Work out the finished part from the listing and answer in its coordinate system (mm). A direction names the side the tool comes from. Round coordinates to 2 decimals unless told otherwise and drop trailing zeros. Write each loop counter-clockwise with the first axis right and the second up, starting at its lowest first coordinate (ties: lowest second). Pieces come first, ordered by that corner, then holes. Notation, with made-up numbers: (-9.75, 48) -> (33.25, 48) arc R28 ccw to (33.25, 82) -> close; hole circle Ø6 at (78.5, 42.25). An arc over 180 degrees is marked (long way). One line per question, with ' | ' between items. Start each with the question number.
```python
from build123d import *

# Parameters (mm, degrees)
F0_W     = 350
F0_H     = 350
F1_DEPTH = 16
F2_DEPTH = 3
F3_W     = 350
F3_H     = 350
F3_W_2   = 318
F3_H_2   = 318
F4_DEPTH = 5
F5_R     = 1


with BuildPart() as f1:
    # F0 (on Front) → F1 (new body)
    with BuildSketch(Plane.XZ):
        with Locations((7.3111886159, -13.1394357215)):
            Rectangle(F0_W, F0_H)
        with BuildLine():
            ThreePointArc((-127.6888113841, 89.8605642785), (-118.3162283821, 112.4879812765), (-95.6888113841, 121.8605642785))
            Line((-95.6888113841, 121.8605642785), (110.3111886159, 121.8605642785))
            ThreePointArc((110.3111886159, 121.8605642785), (132.9386056138, 112.4879812765), (142.3111886159, 89.8605642785))
            Line((142.3111886159, 89.8605642785), (142.3111886159, -116.1394357215))
            ThreePointArc((142.3111886159, -116.1394357215), (132.9386056138, -138.7668527195), (110.3111886159, -148.1394357215))
            Line((110.3111886159, -148.1394357215), (-95.6888113841, -148.1394357215))
            ThreePointArc((-95.6888113841, -148.1394357215), (-118.3162283821, -138.7668527195), (-127.6888113841, -116.1394357215))
            Line((-127.6888113841, -116.1394357215), (-127.6888113841, 89.8605642785))
        make_face(mode=Mode.SUBTRACT)
    extrude(amount=F1_DEPTH)

    # F0 (on Front) → F2 (join)
    with BuildSketch(Plane.XZ):
        with Locations((7.3111886159, -13.1394357215)):
            Rectangle(F0_W, F0_H)
        with BuildLine():
            ThreePointArc((-127.6888113841, 89.8605642785), (-118.3162283821, 112.4879812765), (-95.6888113841, 121.8605642785))
            Line((-95.6888113841, 121.8605642785), (110.3111886159, 121.8605642785))
            ThreePointArc((110.3111886159, 121.8605642785), (132.9386056138, 112.4879812765), (142.3111886159, 89.8605642785))
            Line((142.3111886159, 89.8605642785), (142.3111886159, -116.1394357215))
            ThreePointArc((142.3111886159, -116.1394357215), (132.9386056138, -138.7668527195), (110.3111886159, -148.1394357215))
            Line((110.3111886159, -148.1394357215), (-95.6888113841, -148.1394357215))
            ThreePointArc((-95.6888113841, -148.1394357215), (-118.3162283821, -138.7668527195), (-127.6888113841, -116.1394357215))
            Line((-127.6888113841, -116.1394357215), (-127.6888113841, 89.8605642785))
        make_face(mode=Mode.SUBTRACT)
        with BuildLine():
            Line((110.3111886159, 121.8605642785), (-95.6888113841, 121.8605642785))
            ThreePointArc((-95.6888113841, 121.8605642785), (-118.3162283821, 112.4879812765), (-127.6888113841, 89.8605642785))
            Line((-127.6888113841, 89.8605642785), (-127.6888113841, -116.1394357215))
            ThreePointArc((-127.6888113841, -116.1394357215), (-118.3162283821, -138.7668527195), (-95.6888113841, -148.1394357215))
            Line((-95.6888113841, -148.1394357215), (110.3111886159, -148.1394357215))
            ThreePointArc((110.3111886159, -148.1394357215), (132.9386056138, -138.7668527195), (142.3111886159, -116.1394357215))
            Line((142.3111886159, -116.1394357215), (142.3111886159, 89.8605642785))
            ThreePointArc((142.3111886159, 89.8605642785), (132.9386056138, 112.4879812765), (110.3111886159, 121.8605642785))
        make_face()
    extrude(amount=-F2_DEPTH)

    # F3 (on face) → F4 (join)
    with BuildSketch(Plane(origin=(0, 3, 0), x_dir=(-1, 0, 0), z_dir=(0, 1, 0))):
        with Locations((-7.3111886159, -13.1394357215)):
            Rectangle(F3_W, F3_H)
        with Locations((-7.3111886159, -13.1394357215)):
            Rectangle(F3_W_2, F3_H_2, mode=Mode.SUBTRACT)
    extrude(amount=F4_DEPTH)

    # F5
    f5_edges = [f1.edges().sort_by_distance(p)[0] for p in [
        (7.311189, -16, 161.860564),
        (-167.688811, -16, -13.139436),
        (7.311189, -16, -188.139436),
        (182.311189, -16, -13.139436),
        (-118.316228, -16, 112.487981),
        (7.311189, -16, 121.860564),
        (132.938606, -16, 112.487981),
        (142.311189, -16, -13.139436),
        (132.938606, -16, -138.766853),
        (7.311189, -16, -148.139436),
        (-118.316228, -16, -138.766853),
        (-127.688811, -16, -13.139436),
    ]]
    fillet(f5_edges, radius=F5_R)


solid = f1.part
```
(1) A cutting plane is placed at D-D, the plane x = 79.5. Determine the outline of the cut face in (y, z), then the cut area to 3 significant figures.
(2) A cutting plane is placed at B-B, the plane z = -37.5. Determine the outline of the cut face in (x, y).
(3) For faces 5 (the cylindrical face through (132.688, -7.395, 112.735)), 6 (the flat face through (21, 8, -181)), determine the directions among +Z, -Z, +X, -X, +Y, -Y from which every point of the face is accessible in a straight line to the end or side of a thin tool.
(4) The mould has two halves that part along Z. Classify faces 1 (the flat face through (142.311, -7, -12)), 2 (the flat face through (10, -4, -188.139)), 3 (the flat face through (182.311, -4, -16)), 4 (the flat face through (5, 3, -11)): +Z half, -Z half, draft (parallel to the pull), parting line (faces both ways), or undercut.
(5) A cutting plane is placed at A-A, the plane y = -10. Determine the outline of the cut face in (x, z), then the cut area to 3 significant figures.
(6) Given pin 1 Ø8 at (x, z) = (50.5, 117) entering from +Y; pin 2 Ø1 at (x, z) = (-127.5, -24) entering from -Y, each flat-ended and moving along its own axis, determine where each tip first touches the part or whether it passes through.
(7) Consider L1, parallel to X at y = -13.75, z = 76; L2, parallel to Z at x = 76, y = -5; L3, parallel to Z at x = 33.5, y = 4. Determine where each line is inside the solid, lowest interval first.
(8) A cutting plane is placed at C-C, the plane x = -136. Determine the outline of the cut face in (y, z), then the cut area to 3 significant figures.
Returned:
1) outline: (-16, -187.14) arc R1 ccw to (-15, -188.14) -> (8, -188.14) -> (8, -172.14) -> (3, -172.14) -> (3, 145.86) -> (8, 145.86) -> (8, 161.86) -> (-15, 161.86) arc R1 ccw to (-16, 160.86) -> (-16, 122.86) arc R1 ccw to (-15, 121.86) -> (0, 121.86) -> (0, -148.14) -> (-15, -148.14) arc R1 ccw to (-16, -149.14) -> close | area: 2,490 mm2
2) outline: (-167.69, -15) arc R1 ccw to (-166.69, -16) -> (-128.69, -16) arc R1 ccw to (-127.69, -15) -> (-127.69, 0) -> (142.31, 0) -> (142.31, -15) arc R1 ccw to (143.31, -16) -> (181.31, -16) arc R1 ccw to (182.31, -15) -> (182.31, 8) -> (166.31, 8) -> (166.31, 3) -> (-151.69, 3) -> (-151.69, 8) -> (-167.69, 8) -> close
3) face 5: -Y | face 6: +Z, -Z, +X, -X, +Y
4) face 1: undercut | face 2: -Z half | face 3: draft | face 4: undercut
5) outline: (-167.69, -188.14) -> (182.31, -188.14) -> (182.31, 161.86) -> (-167.69, 161.86) -> close; hole (-127.69, -116.14) arc R32 ccw to (-95.69, -148.14) -> (110.31, -148.14) arc R32 ccw to (142.31, -116.14) -> (142.31, 89.86) arc R32 ccw to (110.31, 121.86) -> (-95.69, 121.86) arc R32 ccw to (-127.69, 89.86) -> close | area: 50,500 mm2
6) pin 1: y = 3 | pin 2: y = -15.72
7) L1: -167.69 to -127.69, 142.31 to 182.31 | L2: -188.14 to -148.14, 121.86 to 161.86 | L3: -188.14 to -172.14, 145.86 to 161.86
8) outline: (-16, -187.14) arc R1 ccw to (-15, -188.14) -> (8, -188.14) -> (8, -172.14) -> (3, -172.14) -> (3, 145.86) -> (8, 145.86) -> (8, 161.86) -> (-15, 161.86) arc R1 ccw to (-16, 160.86) -> close | area: 6,810 mm2
